from build123d import *

# Parameters (mm, degrees)
F1_DEPTH = 4


with BuildPart() as f1:
    # F0 (on Front) → F1 (new body)
    with BuildSketch(Plane.XZ):
        Polygon((0, 6.928203), (-6, 3.464102), (-6, -3.464102), (0, -6.928203), (6, -3.464102), (6, 3.464102), align=None)
    extrude(amount=F1_DEPTH)

    # F2 (on Top) → F3 (revolve, cut)
    with BuildSketch(Plane.XY):
        Polygon((15.133317, 1.273123), (6, -4), (15.133317, -4), align=None)
    revolve(axis=Axis((0, -1.59565, 0), (0, 1, 0)), mode=Mode.SUBTRACT)


solid = f1.part
Can you work these out from the model? Positions are in its coordinate system, mm. Give positions to 0.01 mm unless a question says otherwise; leave off trailing zeros. Write each loop counter-clockwise with the first axis right and the second up, starting at its lowest first coordinate (ties: lowest second). Pieces come first, ordered by that corner, then holes. Notation, with made-up numbers: (49, -39.5) -> (87, -39.5) arc R25 ccw to (87, -10.5) -> close; hole circle Ø9 at (34, 7). An arc over 180 degrees is marked (long way). Answer as a JSON object with one key per item and string values. Group by question number.
Item 1: I'm going to push flat-ended pins straight in: P1, Ø2, axis at x = -3, y = -0.5, coming from the -Z side; P2, Ø2, axis at x = 4.5, y = -2, coming from the +Z side. Where does each tip first touch, or does it pass through?
Item 2: We'd pull the mould along Z, two halves only. Please class faces 1 (the face through (3.042, -1.972, 5.172)), 2 (the face through (2.96, -1.97, -5.22)), 3 (the face through (6, -2, 0)): +Z half, -Z half, draft (parallel to the pull), parting line (faces both ways), or undercut.
Item 3: Suppose I cut it at A-A (y = -1.9). Please give me the cut outline in (x, z), plus the area to 3 significant figures.
Item 4: Please list where these lines run through material, in increasing order: line 1 (Z direction, x = -3, y = -2.5); line 2 (X direction, y = -1.55, z = -4); line 3 (Z direction, x = 4.25, y = -0.15). Write a range as [from, to].
Findings:
{
 "1": {"P1": "stops at z = -5.77", "P2": "stops at z = 4.91"},
 "2": {"face 1": "+Z half", "face 2": "-Z half", "face 3": "draft"},
 "3": {"outline": "(-6, -3.46) -> (0, -6.93) -> (6, -3.46) -> (6, 3.46) -> (0, 6.93) -> (-6, 3.46) -> close", "area": "125 mm²"},
 "4": {"line 1": "z = [-5.2, 5.2]", "line 2": "x = [-5.07, 5.07]", "line 3": "z = [-4.47, 4.47]"}
}
